```python
from build123d import *

# Parameters (mm, degrees)
SKETCH1_W           = 38
SKETCH1_H           = 38
BOSS_EXTRUDE1_DEPTH = 36
SKETCH3_R           = 7
CUT_EXTRUDE1_DEPTH  = 2
FILLET1_R           = 5
FILLET2_R           = 1


with BuildPart() as part:
    # Sketch1 → Boss-Extrude1 (new body)
    with BuildSketch(Plane(origin=(0, 0, 0), x_dir=(1, 0, 0), z_dir=(0, 1, 0))):
        Rectangle(SKETCH1_W, SKETCH1_H)
    extrude(amount=BOSS_EXTRUDE1_DEPTH)

    # Sketch3 → Cut-Extrude1 (cut)
    with BuildSketch(Plane.XZ):
        with Locations(Location((0, 0, 0), (0, 0, 270))):
            Circle(SKETCH3_R)
    extrude(amount=-CUT_EXTRUDE1_DEPTH, mode=Mode.SUBTRACT)

    # Fillet1
    fillet1_edges = [part.edges().sort_by_distance(p)[0] for p in [
        (19, 18, 19),
        (-19, 18, 19),
        (-19, 18, -19),
        (19, 18, -19),
    ]]
    fillet(fillet1_edges, radius=FILLET1_R)

    # Fillet2
    fillet2_edges = [part.edges().sort_by_distance(p)[0] for p in [
        (0, 0, -19),
        (0, 36, -19),
        (19, 0, 0),
        (0, 0, 19),
        (-19, 0, 0),
        (-17.535533906, 0, 17.535533906),
        (-17.535533906, 0, -17.535533906),
        (17.535533906, 0, 17.535533906),
        (17.535533906, 0, -17.535533906),
        (19, 36, 0),
        (-19, 36, 0),
        (0, 36, 19),
        (-17.535533906, 36, 17.535533906),
        (-17.535533906, 36, -17.535533906),
        (17.535533906, 36, 17.535533906),
        (17.535533906, 36, -17.535533906),
    ]]
    fillet(fillet2_edges, radius=FILLET2_R)


solid = part.part
```
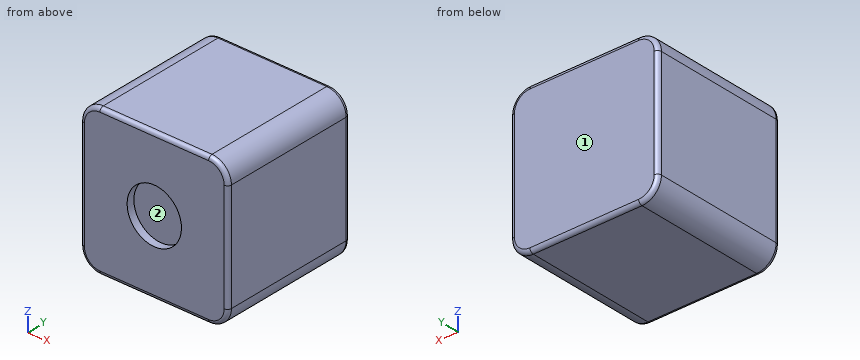
Work out the finished part from the listing and answer in its coordinate system (mm). Face numbers are marked on the shaded views. A direction names the side the tool comes from. Give positions to 0.01 mm unless a question says otherwise; leave off trailing zeros. Loops run counter-clockwise (first coordinate to the right, second up) from the corner with the lowest first, then second, coordinate; pieces in that order, holes last. Notation, with made-up numbers: (58, 35.5) -> (100, 35.5) arc R24 cw to (100, 58.5) -> close; hole circle Ø5 at (-6.5, 52). An arc over 180 degrees is marked (long way). Write item = value, one per line. Start each with the question number.
(1) Which of the six approach directions +Z, -Z, +X, -X, +Y, -Y give full straight-line access (tool end or side, diameter ignored) to the marked faces 1 and 2?
(2) Find the intervals of material crossed by probe 1 along X at (y, z) = (11, -17); probe 2 along X at (y, z) = (0.7, 0); probe 3 along X at (y, z) = (0.5, 0), in increasing order. Write a range as from..to.
(3) Find section A-A on z = 0. Give the vertices of the cut face in (x, y), and give its area (3 significant figures).
(4) Find section B-B on x = 0. Give the vertices of the cut face in (y, z).
From the geometry:
q1.face_1 = +Z, -Z, +X, -X, +Y
q1.face_2 = -Y
q2.probe_1 = -18..18
q2.probe_2 = -18.95..-7, 7..18.95
q2.probe_3 = -18.87..-7, 7..18.87
q3.outline = (-19, 1) arc R1 ccw to (-18, 0) -> (-7, 0) -> (-7, 2) -> (7, 2) -> (7, 0) -> (18, 0) arc R1 ccw to (19, 1) -> (19, 35) arc R1 ccw to (18, 36) -> (-18, 36) arc R1 ccw to (-19, 35) -> close
q3.area = 1,340 mm^2
q4.outline = (0, -18) arc R1 ccw to (1, -19) -> (35, -19) arc R1 ccw to (36, -18) -> (36, 18) arc R1 ccw to (35, 19) -> (1, 19) arc R1 ccw to (0, 18) -> (0, 7) -> (2, 7) -> (2, -7) -> (0, -7) -> close
